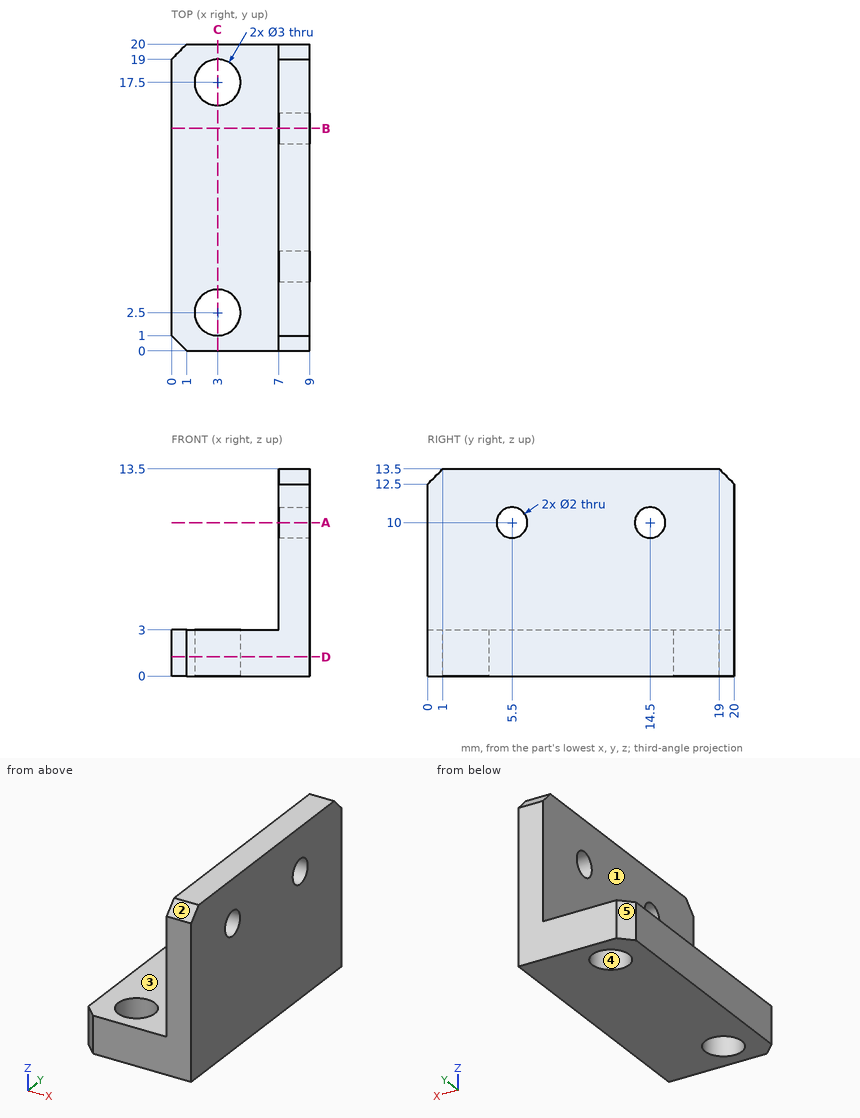
The drawing under review shows one solid part. Ordinate dimensions are in mm from its lowest x, y, z. A direction names the side the tool comes from. Round coordinates to 2 decimals unless told otherwise and drop trailing zeros. Loops run counter-clockwise (first coordinate to the right, second up) from the corner with the lowest first, then second, coordinate; pieces in that order, holes last. Notation, with made-up numbers: (74, 0.25) -> (132, 0.25) arc R17 cw to (132, 4.25) -> close; hole circle Ø9 at (-18.5, -1.5). An arc over 180 degrees is marked (long way). One line per question, with ' | ' between items. Start each with the question number.
Item 1: Draft analysis for pull direction X (two halves, no side actions). For the marked faces 3, 4 and 5, state which applies: +X half, -X half, draft (parallel to the pull), parting line (faces both ways), or undercut.
Item 2: Add section D-D, the plane z = 1.25. Write out the cut boundary in (x, y), then the cut area to 3 significant figures.
Item 3: Wall thickness on line 1 along Y through (x, z) = (3, 1.7); line 2 along Z through (x, y) = (7.65, 14.5); line 3 along Z through (x, y) = (6.5, 7.75): over which ranges is each line inside the solid? List them lowest first. Write a range as [from, to].
Item 4: Add section C-C, the plane x = 3. Write out the cut boundary in (y, z), then the cut area to 3 significant figures.
Item 5: Add section A-A, the plane z = 10. Write out the cut boundary in (x, y).
Item 6: Add section B-B, the plane y = 14.5. Write out the cut boundary in (x, z).
Item 7: For pin 1 (1.8 mm diameter, centred on x = 3, y = 17.5, fed in from +Z); pin 2 (8 mm diameter, centred on y = 6.5, z = 10.5, fed in from -X); pin 3 (2 mm diameter, centred on x = 3, y = 6, fed in from +Z); pin 4 (3 mm diameter, centred on y = 14.5, z = 10, fed in from +X), all flat-tipped, find the tip position at first contact; note any pin that passes through.
Item 8: Machinability: for the marked faces 1 and 2, which of the approach directions +Z, -Z, +X, -X, +Y, -Y give a long, thin tool a straight path to every point of the face, cutting with its end or side? Answer none if there is none.
Return value:
1) face 3: draft | face 4: undercut | face 5: -X half
2) outline: (0, 1) -> (1, 0) -> (9, 0) -> (9, 20) -> (1, 20) -> (0, 19) -> close; hole circle Ø3 at (3, 2.5); hole circle Ø3 at (3, 17.5) | area: 165 mm2
3) line 1: y = [0, 1], [4, 16], [19, 20] | line 2: z = [0, 9], [11, 13.5] | line 3: z = [0, 3]
4) outline: (0, 0) -> (1, 0) -> (1, 3) -> (0, 3) -> close; (4, 0) -> (16, 0) -> (16, 3) -> (4, 3) -> close; (19, 0) -> (20, 0) -> (20, 3) -> (19, 3) -> close | area: 42.0 mm2
5) outline: (7, 0) -> (9, 0) -> (9, 4.5) -> (7, 4.5) -> close; (7, 6.5) -> (9, 6.5) -> (9, 13.5) -> (7, 13.5) -> close; (7, 15.5) -> (9, 15.5) -> (9, 20) -> (7, 20) -> close
6) outline: (0, 0) -> (9, 0) -> (9, 9) -> (7, 9) -> (7, 3) -> (0, 3) -> close; (7, 11) -> (9, 11) -> (9, 13.5) -> (7, 13.5) -> close
7) pin 1: passes through | pin 2: stops at x = 7 | pin 3: stops at z = 3 | pin 4: stops at x = 9
8) face 1: +Z, -X, +Y, -Y | face 2: +Z, +X, -X, -Y
